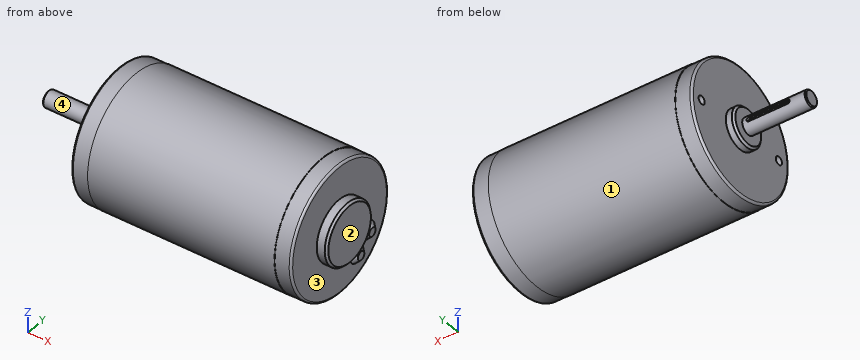
```python
from build123d import *

# Parameters (mm, degrees)
SKETCH1_W                       = 93.1408
SKETCH1_H                       = 32.004
SKETCH2_R                       = 31.877
BOSS_EXTRUDE1_DEPTH             = 8.2296
SKETCH3_R                       = 15.0368
BOSS_EXTRUDE2_DEPTH             = 3.984
SKETCH4_R                       = 15.0368
BOSS_EXTRUDE3_DEPTH             = 1.016
BOSS_EXTRUDE3_TAPER             = 45
SKETCH5_R                       = 31.877
BOSS_EXTRUDE4_DEPTH             = 8.2296
SKETCH6_R                       = 9.525
BOSS_EXTRUDE5_DEPTH             = 4
SKETCH7_R                       = 4
BOSS_EXTRUDE6_DEPTH             = 31.6
CUT_EXTRUDE1_REACH              = 31.204
F_21_0_159_DIAMETER_HOLE1_D     = 4.0386
F_21_0_159_DIAMETER_HOLE1_DEPTH = 13.6144
F_21_0_159_DIAMETER_HOLE1_TIP   = 1.213317848
CHAMFER1_SIZE                   = 1.016
CHAMFER2_SIZE                   = 0.5
FILLET1_R                       = 1


with BuildPart() as part:
    # Sketch1 → Revolve1 (revolve)
    with BuildSketch(Plane.XY):
        with Locations((54.8, 16.002)):
            Rectangle(SKETCH1_W, SKETCH1_H)
    revolve(axis=Axis((8.2296, 0, 0), (1, 0, 0)))

    # Sketch2 → Boss-Extrude1 (add)
    with BuildSketch(Plane(origin=(101.3704, 0, 0), x_dir=(0, 0, -1), z_dir=(1, 0, 0))):
        Circle(SKETCH2_R)
    extrude(amount=BOSS_EXTRUDE1_DEPTH)

    # Sketch3 → Boss-Extrude2 (add)
    with BuildSketch(Plane(origin=(109.6, 0, 0), x_dir=(0, 0, -1), z_dir=(1, 0, 0))):
        Circle(SKETCH3_R)
    extrude(amount=BOSS_EXTRUDE2_DEPTH)

    # Sketch4 → Boss-Extrude3 (add)
    with BuildSketch(Plane(origin=(113.584, 0, 0), x_dir=(0, 0, -1), z_dir=(1, 0, 0))):
        Circle(SKETCH4_R)
    extrude(amount=BOSS_EXTRUDE3_DEPTH, taper=BOSS_EXTRUDE3_TAPER)

    # Sketch5 → Boss-Extrude4 (add)
    with BuildSketch(Plane.ZY.offset(-8.2296)):
        Circle(SKETCH5_R)
    extrude(amount=BOSS_EXTRUDE4_DEPTH)

    # Sketch6 → Boss-Extrude5 (add)
    with BuildSketch(Plane.ZY):
        Circle(SKETCH6_R)
    extrude(amount=BOSS_EXTRUDE5_DEPTH)

    # Sketch7 → Boss-Extrude6 (add)
    with BuildSketch(Plane.ZY.offset(4)):
        Circle(SKETCH7_R)
    extrude(amount=BOSS_EXTRUDE6_DEPTH)

    # Sketch8 → Cut-Extrude1 (cut, up to next)
    with BuildSketch(Plane.XZ.offset(-2.8), mode=Mode.PRIVATE) as cut_extrude1_sk1:
        with BuildLine():
            Line((-7.1, 1), (-26.6, 1))
            ThreePointArc((-26.6, 1), (-27.6, 0), (-26.6, -1))
            Line((-26.6, -1), (-7.1, -1))
            ThreePointArc((-7.1, -1), (-6.1, 0), (-7.1, 1))
        make_face()
    cut_extrude1_tool1 = extrude(cut_extrude1_sk1.sketch, amount=-CUT_EXTRUDE1_REACH, mode=Mode.PRIVATE) & part.part
    add(cut_extrude1_tool1.solids().sort_by_distance((-16.85, 2.8, 0))[0], mode=Mode.SUBTRACT)

    # Sketch9 → Revolve2 (revolve)
    with BuildSketch(Plane.XY.offset(-18.607090683)):
        Polygon((109.6, 15.525359639), (109.6, 11.207359639), (111.8479, 11.207359639), (111.8479, 13.325359639), (109.6479, 15.525359639), align=None)
    revolve(axis=Axis((109.6, 11.207359639, -18.607090683), (1, 0, 0)))

    # Sketch10 → Revolve3 (revolve)
    with BuildSketch(Plane.XY.offset(-11.207359639)):
        Polygon((109.6, 22.925090683), (109.6, 18.607090683), (111.8479, 18.607090683), (111.8479, 20.725090683), (109.6479, 22.925090683), align=None)
    revolve(axis=Axis((109.6, 18.607090683, -11.207359639), (1, 0, 0)))

    # #21 (0.159) Diameter Hole1
    with Locations(Plane.ZY):
        with Locations((0, 25.4), (0, -25.4)):
            Hole(F_21_0_159_DIAMETER_HOLE1_D / 2, depth=F_21_0_159_DIAMETER_HOLE1_DEPTH)
            with Locations((0, 0, -(F_21_0_159_DIAMETER_HOLE1_DEPTH + F_21_0_159_DIAMETER_HOLE1_TIP / 2))):  # 118° drill point
                Cone(0, F_21_0_159_DIAMETER_HOLE1_D / 2, F_21_0_159_DIAMETER_HOLE1_TIP, mode=Mode.SUBTRACT)

    # Chamfer1
    chamfer1_edges = [part.edges().sort_by_distance(p)[0] for p in [
        (-4, 0, -9.525),
    ]]
    chamfer(chamfer1_edges, length=CHAMFER1_SIZE)

    # Chamfer2
    chamfer2_edges = [part.edges().sort_by_distance(p)[0] for p in [
        (-35.6, 0, -4),
    ]]
    chamfer(chamfer2_edges, length=CHAMFER2_SIZE)

    # Fillet1
    fillet1_edges = [part.edges().sort_by_distance(p)[0] for p in [
        (0, 0, -31.877),
        (109.6, 0, 31.877),
    ]]
    fillet(fillet1_edges, radius=FILLET1_R)


solid = part.part
```
Part model, mm, in its own coordinate system. Face numbers are marked on the shaded views. A direction names the side the tool comes from. Coordinates: 2 decimals unless noted, no trailing zeros. Loops run counter-clockwise (first coordinate to the right, second up) from the corner with the lowest first, then second, coordinate; pieces in that order, holes last. Notation, with made-up numbers: (40, 35) - (95, 35) arc R11 cw to (95, 52) - close; hole circle Ø8 at (21.25, 13). An arc over 180 degrees is marked (long way). Write item = value, one per line. Start each with the question number.
Item 1: Flat gauge pins, fed straight in: pin 1 Ø1 at (x, z) = (66, 4.5) entering from +Y; pin 2 Ø4 at (x, y) = (38.5, -10) entering from +Z; pin 3 Ø1.2 at (x, y) = (-14.5, 3.5) entering from +Z (3 decimals). Where does each tip first touch, or does it go through?
Item 2: 3-axis set-ups, long thin cutter, end or side, ignore diameter. For the marked faces 3 and 4: which of +Z, -Z, +X, -X, +Y, -Y reach the whole face in a straight line?
Item 3: Mould opens along Z. For the marked faces 1 and 2 say: released by +Z, released by -Z, zero draft, split by the parting line, or undercut.
Item 4: Cut at A-A, the plane x = 4. Give the cut face in (y, z), and give its area (3 significant figures).
Item 5: Wall check: L1, parallel to Y at x = 6.75, z = 0; L2, parallel to X at y = 13, z = -5; L3, parallel to Z at x = 6, y = 25. Give the ranges that are in metal, low to high. Write a range as from..to.
Item 6: Cut at B-B, the plane x = 94. Give the cut face in (y, z), and give its area (3 significant figures).
The answers:
q1.pin_1 = 31.75
q1.pin_2 = 30.99
q1.pin_3 = 2.755
q2.face_3 = +X
q2.face_4 = -X
q3.face_1 = split by the parting line
q3.face_2 = zero draft
q4.outline = circle Ø63.75 at (0, 0); hole circle Ø4.04 at (-25.4, 0); hole circle Ø4.04 at (25.4, 0)
q4.area = 3,170 mm2
q5.L1 = -31.88..-27.42, -23.38..23.38, 27.42..31.88
q5.L2 = 0..114.6
q5.L3 = -19.78..-1.98, 1.98..19.78
q6.outline = circle Ø64.01 at (0, 0)
q6.area = 3,220 mm2
